from build123d import *

# Parameters (mm, degrees)
SKETCH1_R           = 2
BOSS_EXTRUDE1_DEPTH = 5
FILLET1_R           = 5


with BuildPart() as part:
    # Sketch1 → Boss-Extrude1 (new body)
    with BuildSketch(Plane.XY):
        with BuildLine():
            Line((-29.613436562, 8), (-18.33030278, 8))
            ThreePointArc((-18.33030278, 8), (-12.975595941, 15.219523973), (-5, 19.364916731))
            Line((-5, 19.364916731), (5, 19.364916731))
            ThreePointArc((5, 19.364916731), (12.975595941, 15.219523973), (18.33030278, 8))
            Line((18.33030278, 8), (29.613436562, 8))
            ThreePointArc((29.613436562, 8), (22.00766613, 21.368627857), (8.868894541, 29.364916731))
            Line((8.868894541, 29.364916731), (-8.868894541, 29.364916731))
            ThreePointArc((-8.868894541, 29.364916731), (-22.00766613, 21.368627857), (-29.613436562, 8))
        make_face()
        with Locations((20.784609691, 12)):
            Circle(SKETCH1_R, mode=Mode.SUBTRACT)
        with Locations((-20.784609691, 12)):
            Circle(SKETCH1_R, mode=Mode.SUBTRACT)
        with Locations((-5, 24.364916731)):
            Circle(SKETCH1_R, mode=Mode.SUBTRACT)
        with Locations(Location((5, 24.364916731, 0), (0, 0, 180))):
            Circle(SKETCH1_R, mode=Mode.SUBTRACT)
    extrude(amount=BOSS_EXTRUDE1_DEPTH)

    # Fillet1
    fillet1_edges = [part.edges().sort_by_distance(p)[0] for p in [
        (-18.33030278, 8, 2.5),
        (-29.613436562, 8, 2.5),
        (-8.868894541, 29.364916731, 2.5),
        (8.868894541, 29.364916731, 2.5),
        (29.613436562, 8, 2.5),
        (18.33030278, 8, 2.5),
        (5, 19.364916731, 2.5),
        (-5, 19.364916731, 2.5),
    ]]
    fillet(fillet1_edges, radius=FILLET1_R)


solid = part.part
Model file for the job. Use its own axes, mm. A direction names the side the tool comes from. Round coordinates to 2 decimals unless told otherwise and drop trailing zeros. Loops run counter-clockwise (first coordinate to the right, second up) from the corner with the lowest first, then second, coordinate; pieces in that order, holes last.
1. Band-saw the part on D-D, the plane y = 28.25. List the corners of the cut face in (x, z).
Check values:
outline: (-11.95, 0) - (11.95, 0) - (11.95, 5) - (-11.95, 5) - close
2. Drop flat-ended pins along their axis: P1, Ø6.5, axis at x = -20.78, y = 12, coming from the -Z side; P2, Ø2, axis at y = 22.5, z = 1.5, coming from the +X side; P3, Ø3, axis at x = -17.5, z = 1.5, coming from the +Y side; P4, Ø1.5, axis at x = 0, z = 2, coming from the -Y side. Give the stop position or say it passes through.
Check values:
P1: stops at z = 0
P2: stops at x = 21.88
P3: stops at y = 26.17
P4: stops at y = 19.36
3. Tool access for faces 4 (the cylindrical face through (-8.9, 29.3, 2.5)), 5 (the cylindrical face through (5.036, 19.313, 2.535)): list every direction of +Z, -Z, +X, -X, +Y, -Y with a clear straight run to the whole face (end or side of a thin tool).
Check values:
face 4: +Z, -Z, -X, +Y
face 5: +Z, -Z, -Y
4. Band-saw the part on A-A, the plane y = 12. List the corners of the cut face in (x, z), and give its area (3 significant figures).
Check values:
outline: (-27.04, 0) - (-22.78, 0) - (-22.78, 5) - (-27.04, 5) - close; (-18.78, 0) - (-16, 0) - (-16, 5) - (-18.78, 5) - close; (16, 0) - (18.78, 0) - (18.78, 5) - (16, 5) - close; (22.78, 0) - (27.04, 0) - (27.04, 5) - (22.78, 5) - close
area: 70.4 mm2
5. Wall check: probe 1 along X at (y, z) = (26, 3.3); probe 2 along X at (y, z) = (23.5, 2.6); probe 3 along X at (y, z) = (10.5, 2.2). Give the ranges that are in metal, low to high.
Check values:
probe 1: x = -16.28 to -6.15, -3.85 to 3.85, 6.15 to 16.28
probe 2: x = -19.72 to -6.8, -3.2 to 3.2, 6.8 to 19.72
probe 3: x = -26.47 to -22.11, -19.46 to -17.02, 17.02 to 19.46, 22.11 to 26.47
6. Mould opens along Z. For faces 1 (the cylindrical face through (-22.26, 13.35, 2.46)), 2 (the flat face through (0, 21, 5)), 3 (the flat face through (0, 21, 0)) say: +Z half, -Z half, draft (parallel to the pull), parting line (faces both ways), or undercut.
Check values:
face 1: draft
face 2: +Z half
face 3: -Z half
7. Band-saw the part on C-C, the plane z = 2.85. List the corners of the cut face in (x, y) (3 decimals).
Check values:
outline: (-26.452, 15.532) arc R5 ccw to (-22.141, 8) - (-21.354, 8) arc R5 ccw to (-17.083, 10.4) arc R20 cw to (-5.758, 19.153) arc R5 cw to (-4.318, 19.365) - (4.318, 19.365) arc R5 cw to (5.758, 19.153) arc R20 cw to (17.083, 10.4) arc R5 ccw to (21.354, 8) - (22.141, 8) arc R5 ccw to (26.452, 15.532) arc R30.675 ccw to (9.673, 29.11) arc R5 ccw to (8.097, 29.365) - (-8.097, 29.365) arc R5 ccw to (-9.673, 29.11) arc R30.675 ccw to start; hole circle Ø4 at (-20.785, 12); hole circle Ø4 at (-5, 24.365); hole circle Ø4 at (5, 24.365); hole circle Ø4 at (20.785, 12)
8. Band-saw the part on B-B, the plane x = -5. List the corners of the cut face in (y, z), and give its area (3 significant figures).
Check values:
outline: (19.32, 0) - (22.36, 0) - (22.36, 5) - (19.32, 5) - close; (26.36, 0) - (29.36, 0) - (29.36, 5) - (26.36, 5) - close
area: 30.2 mm2
